Source: CAD feature listing. Evaluate the final solid. Frame: model axes, mm. Face numbers are marked on the shaded views. A direction names the side the tool comes from. Give positions to 0.01 mm unless a question says otherwise; leave off trailing zeros. Loops run counter-clockwise (first coordinate to the right, second up) from the corner with the lowest first, then second, coordinate; pieces in that order, holes last.
from build123d import *

# Parameters (mm, degrees)
SKETCH1_R                  = 12.6
BOSS_EXTRUDE1_DEPTH        = 12
FILLET1_R                  = 5
FILLET2_R                  = 2
F_5_5_5_5_DIAMETER_HOLE1_D = 5.5
FILLET3_R                  = 1
M5_TAPPED_HOLE1_REACH      = 65.765
M5_TAPPED_HOLE1_BORE_R     = 2.1
CHAMFER1_SIZE              = 0.5
CHAMFER2_SIZE              = 1


with BuildPart() as part:
    # Sketch1 → Boss-Extrude1 (new body)
    with BuildSketch(Plane(origin=(0, 0, 0), x_dir=(1, 0, 0), z_dir=(0, 1, 0))):
        with BuildLine():
            Line((-49, 20), (-34, 20))
            Line((-34, 20), (-34, 18.5))
            Line((-34, 18.5), (-22, 18.5))
            Line((-22, 18.5), (-22, 20))
            Line((-22, 20), (22, 20))
            Line((22, 20), (22, 18.5))
            Line((22, 18.5), (34, 18.5))
            Line((34, 18.5), (34, 20))
            Line((34, 20), (49, 20))
            Line((49, 20), (49, 10))
            Line((49, 10), (20, 10))
            Line((20, 10), (20, 0))
            ThreePointArc((20, 0), (16.200308021, -11.728172066), (6.244997998, -19))
            Line((6.244997998, -19), (-6.244997998, -19))
            ThreePointArc((-6.244997998, -19), (-16.200308021, -11.728172066), (-20, 0))
            Line((-20, 0), (-20, 10))
            Line((-20, 10), (-49, 10))
            Line((-49, 10), (-49, 20))
        make_face()
        with Locations(Location((0, 0, 0), (0, 0, 270))):
            Circle(SKETCH1_R, mode=Mode.SUBTRACT)
    extrude(amount=BOSS_EXTRUDE1_DEPTH)

    # Fillet1
    fillet1_edges = [part.edges().sort_by_distance(p)[0] for p in [
        (20, 6, -10),
        (-20, 6, -10),
    ]]
    fillet(fillet1_edges, radius=FILLET1_R)

    # Fillet2
    fillet2_edges = [part.edges().sort_by_distance(p)[0] for p in [
        (49, 6, -10),
        (-49, 6, -10),
    ]]
    fillet(fillet2_edges, radius=FILLET2_R)

    # Ø5.5 (5.5) Diameter Hole1 (through all)
    with Locations(Plane.XY.offset(-10)):
        with Locations((-43.25, 6), (43.25, 6)):
            Hole(F_5_5_5_5_DIAMETER_HOLE1_D / 2)

    # Fillet3
    fillet3_edges = [part.edges().sort_by_distance(p)[0] for p in [
        (-34, 6, -18.5),
        (-22, 6, -18.5),
        (22, 6, -18.5),
        (34, 6, -18.5),
    ]]
    fillet(fillet3_edges, radius=FILLET3_R)

    # M5 Tapped Hole1 bore → M5 Tapped Hole1 (cut, up to next)
    with BuildSketch(Plane.XY.offset(19), mode=Mode.PRIVATE) as m5_tapped_hole1_sk1:
        with Locations((0, 6)):
            Circle(M5_TAPPED_HOLE1_BORE_R)
    m5_tapped_hole1_tool1 = extrude(m5_tapped_hole1_sk1.sketch, amount=-M5_TAPPED_HOLE1_REACH, mode=Mode.PRIVATE) & part.part
    add(m5_tapped_hole1_tool1.solids().sort_by_distance((0, 6, 19))[0], mode=Mode.SUBTRACT)

    # Chamfer1
    chamfer1_edges = [part.edges().sort_by_distance(p)[0] for p in [
        (46, 6, -10),
        (-40.5, 6, -10),
    ]]
    chamfer(chamfer1_edges, length=CHAMFER1_SIZE)

    # Chamfer2
    chamfer2_edges = [part.edges().sort_by_distance(p)[0] for p in [
        (0, 12, -12.6),
    ]]
    chamfer(chamfer2_edges, length=CHAMFER2_SIZE)


solid = part.part
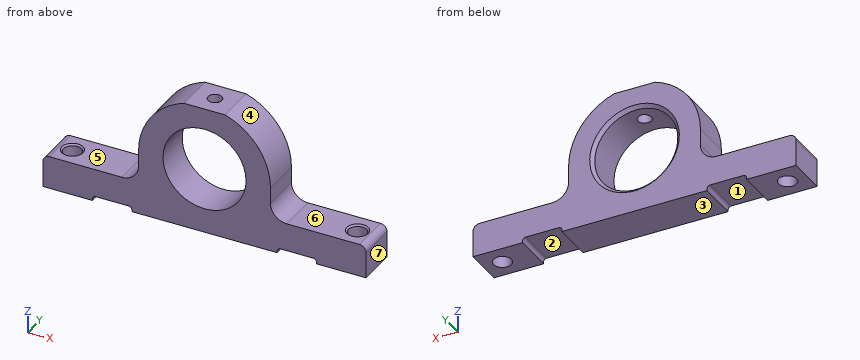
1) Cut plane A-A (x = 0). Return loops of the section in (y, z).
Checks:
outline: (0, -20) - (12, -20) - (12, -13.6) - (11, -12.6) - (0, -12.6) - close; (0, 12.6) - (3.9, 12.6) - (3.9, 19) - (0, 19) - close; (8.1, 12.6) - (11, 12.6) - (12, 13.6) - (12, 19) - (8.1, 19) - close
2) Pull-direction query (X, two-part tool) for the marked faces 1, 2, 3 and 4; classes: released by +X, released by -X, zero draft, split by the parting line, or undercut.
Checks:
face 1: undercut
face 2: undercut
face 3: zero draft
face 4: released by +X
3) Cut plane B-B (x = -43.25). Return loops of the section in (y, z), and give its area (4 significant figures).
Checks:
outline: (0, -20) - (3.25, -20) - (3.25, -10.5) - (2.75, -10) - (0, -10) - close; (8.75, -20) - (12, -20) - (12, -10) - (9.25, -10) - (8.75, -10.5) - close
area: 64.75 mm2
4) Reachability of the marked faces 5, 6 and 7 from +Z, -Z, +X, -X, +Y, -Y: full face, straight path, thin tool, end or side. Return the list, or none.
Checks:
face 5: +Z, -X, +Y, -Y
face 6: +Z, +X, +Y, -Y
face 7: +Z, -Z, +X, +Y, -Y
5) Cut plane D-D (x = 39). Return loops of the section in (y, z), and give its area (3 significant figures).
Checks:
outline: (0, -20) - (12, -20) - (12, -10) - (0, -10) - close
area: 120 mm2
6) Contact query for flat-ended pins moving along their axis: P1, Ø3, axis at x = 29.5, y = 6.5, coming from the -Z side; P2, Ø2.5, axis at y = 8.5, z = -3, coming from the +X side; P3, Ø5, axis at x = -29, y = 5.5, coming from the +Z side. Output: stop coordinate, or through.
Checks:
P1: stops at z = -18.5
P2: stops at x = 20
P3: stops at z = -10
7) Cut plane C-C (y = 6). State how many separate pieces and enclosed holes the cut face has, and give its area (3 significant figures).
Checks:
separate pieces: 3
enclosed holes: 0
area: 1,340 mm2
8) Ray query, probe 1 along X at (y, z) = (7.5, 0); probe 2 along Y at (x, z) = (43.25, -15.5); probe 3 along Z at (x, y) = (29.5, 9.75). Return the intervals inside material, ascending.
Checks:
probe 1: x = -20 to -12.6, 12.6 to 20
probe 2: y = 0 to 3.25, 8.75 to 12
probe 3: z = -18.5 to -10
